The model under review builds one solid part; all positions refer to its coordinate system, in mm. Face numbers are marked on the shaded views. A direction names the side the tool comes from. Give positions to 0.01 mm unless a question says otherwise; leave off trailing zeros. Write each loop counter-clockwise with the first axis right and the second up, starting at its lowest first coordinate (ties: lowest second). Pieces come first, ordered by that corner, then holes. Notation, with made-up numbers: M 33.5,-7.5 L 71.5,-7.5 A23 cw 71.5,21.5 Z; hole C 38,15.25 d6. An arc over 180 degrees is marked long. Write each question's results on one line, items separated by ' | '. Start each with the question number.
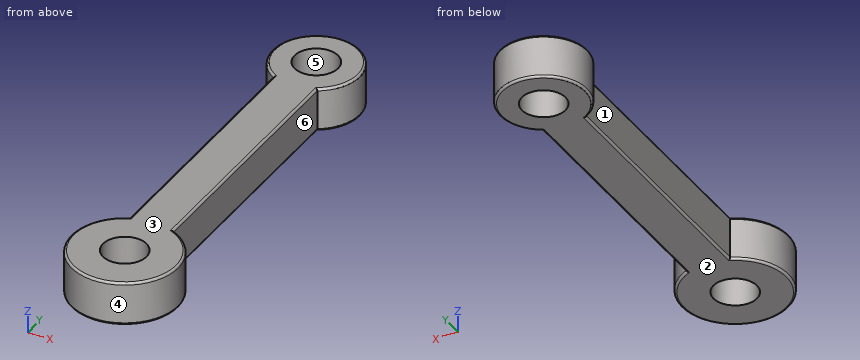
from build123d import *

# Parameters (mm, degrees)
ESQUISSE1_R        = 10
BOSS_EXTRU_1_DEPTH = 20
CONG_2_R           = 1


with BuildPart() as part:
    # Esquisse1 → Boss.-Extru.1 (new body)
    with BuildSketch(Plane.XY):
        with BuildLine():
            Line((-10, -17.320508076), (-10, -137.320508076))
            ThreePointArc((-10, -137.320508076), (0, -184.099247501), (10, -137.320508076))
            Line((10, -137.320508076), (10, -17.320508076))
            ThreePointArc((10, -17.320508076), (0, 20), (-10, -17.320508076))
        make_face()
        Circle(ESQUISSE1_R, mode=Mode.SUBTRACT)
        with Locations((0, -159.641016151)):
            Circle(ESQUISSE1_R, mode=Mode.SUBTRACT)
    extrude(amount=BOSS_EXTRU_1_DEPTH)

    # Congé2
    cong_2_edges = [part.edges().sort_by_distance(p)[0] for p in [
        (0, -184.099247501, 20),
        (10, -77.320508076, 20),
        (0, 20, 20),
        (10, -77.320508076, 0),
        (0, -184.099247501, 0),
        (-10, -77.320508076, 0),
        (0, 20, 0),
        (-10, -77.320508076, 20),
    ]]
    fillet(cong_2_edges, radius=CONG_2_R)


solid = part.part
(1) Wall thickness on L1, parallel to Y at x = 0, z = 8.5; L2, parallel to Y at x = -7, z = 11.75 (3 decimals); L3, parallel to X at y = -91, z = 11.75: over which ranges is each line inside the solid? List them lowest first.
(2) Add section A-A (y = -63.5). State the section outline as (x, z) points, then the cut area to 3 significant figures.
(3) Add section C-C (z = 3.75). State the section outline as (x, y) points, then the cut area to 3 significant figures.
(4) Machinability: for the marked faces 1 and 2, which of the approach directions +Z, -Z, +X, -X, +Y, -Y give a long, thin tool a straight path to every point of the face, cutting with its end or side? Answer none if there is none.
(5) Add section B-B (x = 0). Give the number of separate pieces and of enclosed holes in the cut face, then the cut area to 3 significant figures.
(6) Draft analysis for pull direction X (two halves, no side actions). For the marked faces 3, 4, 5 and 6, state which applies: pulls with the +X half, pulls with the -X half, needs draft (parallel to the pull), parting line crosses it, or undercut.
(7) Clearance check with flat-ended pins moving along their axes: P1, Ø6, axis at x = -16.5, z = 10.5, coming from the +Y side; P2, Ø12, axis at y = -95, z = 6, coming from the +X side; P3, Ø12, axis at x = -14, z = 2.5, coming from the -Y side; P4, Ø6, axis at x = -18.5, y = -135.5, coming from the +Z side. State where each tip first meets the part, or that it passes through.
Calculated:
1) L1: y = -184.1 to -169.64, -149.64 to -10, 10 to 20 | L2: y = -183.076 to -166.782, -152.5 to -7.141, 7.141 to 18.735 | L3: x = -10 to 10
2) outline: M -10,1 A1 ccw -9,0 L 9,0 A1 ccw 10,1 L 10,19 A1 ccw 9,20 L -9,20 A1 ccw -10,19 Z | area: 399 mm²
3) outline: M -10,-137.32 A24.46 ccw long 10,-137.32 L 10,-17.32 A20 ccw long -10,-17.32 Z; hole C 0,-159.64 d20; hole C 0,0 d20 | area: 4,840 mm²
4) face 1: +Z, -Z, -X | face 2: -Z, +X, -X, +Y, -Y
5) separate pieces: 3 | enclosed holes: 0 | area: 3,280 mm²
6) face 3: needs draft | face 4: parting line crosses it | face 5: undercut | face 6: pulls with the +X half
7) P1: stops at y = 14.76 | P2: stops at x = 10 | P3: stops at y = -182.75 | P4: passes through
